```python
from build123d import *

# Parameters (mm, degrees)
F0_W     = 15.24
F0_H     = 6.35
F1_DEPTH = 177.8
F2_R     = 2.3876
F3_DEPTH = 15.241
F4_R     = 15.875
F5_DEPTH = 10.16
F6_R     = 13.97
F7_DEPTH = 8.89


with BuildPart() as f1:
    # F0 (on Front) → F1 (new body)
    with BuildSketch(Plane.XZ):
        with Locations((1.651002, -2.908992)):
            Rectangle(F0_W, F0_H)
    extrude(amount=F1_DEPTH)

    # F2 (on face) → F3 (cut, through all)
    with BuildSketch(Plane.YZ.offset(9.271002)):
        with Locations((-120.65, -2.908992)):
            Circle(F2_R)
    extrude(amount=-F3_DEPTH, mode=Mode.SUBTRACT)

    # F4 (on face) → F5 (join)
    with BuildSketch(Plane.XY.offset(0.266008)):
        with Locations((1.651002, -12.7)):
            Circle(F4_R)
    extrude(amount=F5_DEPTH)

    # F6 (on face) → F7 (cut)
    with BuildSketch(Plane.XY.offset(10.426008)):
        with Locations((1.651002, -12.7)):
            Circle(F6_R)
    extrude(amount=-F7_DEPTH, mode=Mode.SUBTRACT)


solid = f1.part
```
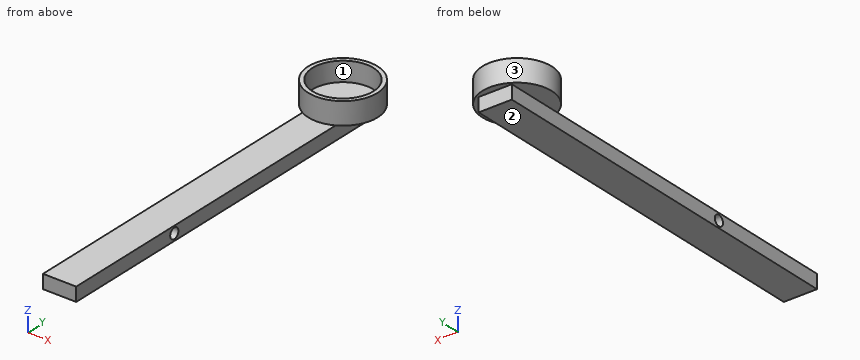
Read the model definition and answer for the solid it produces. Units are mm, in the model's axes. Face numbers are marked on the shaded views. Give positions to 0.01 mm unless a question says otherwise; leave off trailing zeros. Loops run counter-clockwise (first coordinate to the right, second up) from the corner with the lowest first, then second, coordinate; pieces in that order, holes last.
Item 1: The mould has two halves that part along Y. Classify the marked faces 1, 2 and 3: released by +Y, released by -Y, zero draft, split by the parting line, or undercut.
Item 2: Each of these flat-tipped pins is pushed along its axis until it touches: pin 1 Ø1 at (y, z) = (-77, -3) entering from -X; pin 2 Ø8 at (y, z) = (-93.5, 5.5) entering from +X; pin 3 Ø5 at (x, z) = (-0.5, -2) entering from +Y; pin 4 Ø8 at (x, z) = (-8, 5.5) entering from -Y. Where does it stop, or does it pass through?
Item 3: The part is cut by section B-B (y = -12.7). Write down the section's boundary in (x, z).
Item 4: Find the intervals of material crossed by line 1 along Z through (x, y) = (-5.5, -73.5); line 2 along X through (y, z) = (-84, -2); line 3 along Y through (x, z) = (5, 3), in increasing order.
Item 5: The part is cut by section D-D (x = -8). Write down the section's boundary in (y, z), and give its area (3 significant figures).
Item 6: The part is cut by section C-C (z = 6). Write down the section's boundary in (x, y) (3 decimals), and give its area (3 significant figures).
Item 7: The part is cut by section A-A (y = -120.65). Write down the section's boundary in (x, z), and give its area (3 significant figures).
Taken from the geometry:
1. face 1: undercut
1. face 2: zero draft
1. face 3: split by the parting line
2. pin 1: stops at x = -5.97
2. pin 2: passes through
2. pin 3: stops at y = 3.14
2. pin 4: stops at y = -27.54
3. outline: (-14.22, 0.27) - (-5.97, 0.27) - (-5.97, -6.08) - (9.27, -6.08) - (9.27, 0.27) - (17.53, 0.27) - (17.53, 10.43) - (15.62, 10.43) - (15.62, 1.54) - (-12.32, 1.54) - (-12.32, 10.43) - (-14.22, 10.43) - close
4. line 1: z = -6.08 to 0.27
4. line 2: x = -5.97 to 9.27
4. line 3: y = -28.22 to -26.26, 0.86 to 2.82
5. outline: (-25.3, 0.27) - (-0.1, 0.27) - (-0.1, 10.43) - (-2.6, 10.43) - (-2.6, 1.54) - (-22.8, 1.54) - (-22.8, 10.43) - (-25.3, 10.43) - close
5. area: 76.5 mm2
6. outline: circle Ø31.75 at (1.651, -12.7); hole circle Ø27.94 at (1.651, -12.7)
6. area: 179 mm2
7. outline: (-5.97, -6.08) - (9.27, -6.08) - (9.27, -5.3) - (-5.97, -5.3) - close; (-5.97, -0.52) - (9.27, -0.52) - (9.27, 0.27) - (-5.97, 0.27) - close
7. area: 24.0 mm2
